Part model, mm, in its own coordinate system. Face numbers are marked on the shaded views. Coordinates: 2 decimals unless noted, no trailing zeros. Order: outer loops, then holes, each group sorted by start corner. A loop starts at its lowest first (then second) coordinate and runs counter-clockwise, first axis right, second up.
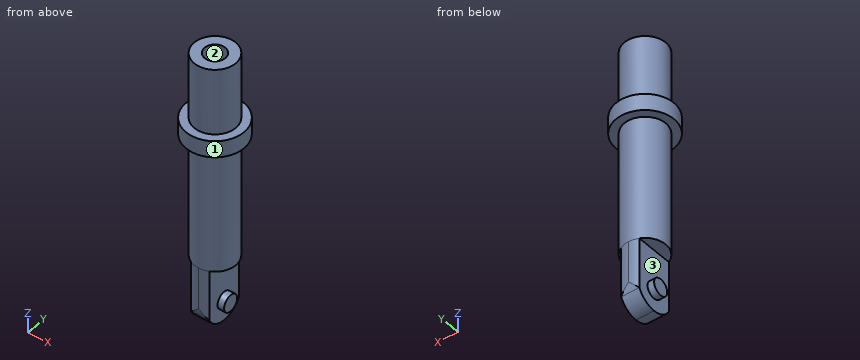
from build123d import *

# Parameters (mm, degrees)
F0_R          = 5
F1_DEPTH      = 50
F3_DEPTH      = 15
F5_DEPTH      = 25
F6_R          = 2
F7_DEPTH      = 1.6
F7_DEPTH_BACK = 6
F8_R          = 2.5
F9_DEPTH      = 10
F11_R         = 7
F11_R_2       = 5
F12_DEPTH     = 4


with BuildPart() as f1:
    # F0 (on Top) → F1 (new body)
    with BuildSketch(Plane.XY):
        Circle(F0_R)
    extrude(amount=F1_DEPTH)

    # F2 (on face) → F3 (join)
    with BuildSketch(Plane(origin=(0, 0, 0), x_dir=(1, 0, 0), z_dir=(0, 0, -1))):
        with BuildLine():
            ThreePointArc((2.2, 4.4899888641), (1.1291713066, 4.8708286934), (0, 5))
            ThreePointArc((0, 5), (-1.1291713066, 4.8708286934), (-2.2, 4.4899888641))
            Line((-2.2, 4.4899888641), (-2.2, -4.4899888641))
            ThreePointArc((-2.2, -4.4899888641), (-1.1291713066, -4.8708286934), (0, -5))
            ThreePointArc((0, -5), (1.1291713066, -4.8708286934), (2.2, -4.4899888641))
            Line((2.2, -4.4899888641), (2.2, 4.4899888641))
        make_face()
    extrude(amount=F3_DEPTH)

    # F4 (on face) → F5 (cut)
    with BuildSketch(Plane.YZ.offset(2.2)):
        with BuildLine():
            Line((5, -15), (5, -10))
            ThreePointArc((5, -10), (4.8708286934, -11.1291713066), (4.4899888641, -12.2))
            Line((4.4899888641, -12.2), (4.4899888641, -15))
            Line((4.4899888641, -15), (5, -15))
        make_face()
        with BuildLine():
            Line((4.4899888641, -15), (4.4899888641, -12.2))
            ThreePointArc((4.4899888641, -12.2), (2.6457513111, -14.2426406871), (0, -15))
            Line((0, -15), (4.4899888641, -15))
        make_face()
        with BuildLine():
            Line((-4.4899888641, -15), (0, -15))
            ThreePointArc((0, -15), (-2.6457513111, -14.2426406871), (-4.4899888641, -12.2))
            Line((-4.4899888641, -12.2), (-4.4899888641, -15))
        make_face()
        with BuildLine():
            ThreePointArc((-4.4899888641, -12.2), (-4.8708286934, -11.1291713066), (-5, -10))
            Line((-5, -10), (-5, -15))
            Line((-5, -15), (-4.4899888641, -15))
            Line((-4.4899888641, -15), (-4.4899888641, -12.2))
        make_face()
    extrude(amount=-F5_DEPTH, mode=Mode.SUBTRACT)

    # F6 (on face) → F7 (join, two sides)
    with BuildSketch(Plane.YZ.offset(2.2)) as f7_sk:
        with Locations((0, -10)):
            Circle(F6_R)
    extrude(amount=F7_DEPTH)
    extrude(f7_sk.sketch, amount=-F7_DEPTH_BACK)

    # F8 (on face) → F9 (cut)
    with BuildSketch(Plane.XY.offset(50)):
        Circle(F8_R)
    extrude(amount=-F9_DEPTH, mode=Mode.SUBTRACT)

    # F11 (on offset) → F12 (join)
    with BuildSketch(Plane.XY.offset(30)):
        Circle(F11_R)
        Circle(F11_R_2, mode=Mode.SUBTRACT)
    extrude(amount=F12_DEPTH)


solid = f1.part
Q1. Wall check: line 1 along Y through (x, z) = (0, 45.5); line 2 along X through (y, z) = (-0.25, 45.5); line 3 along Z through (x, y) = (5.5, 2.25). Give the ranges that are in metal, low to high.
Results list:
line 1: y = -5 to -2.5, 2.5 to 5
line 2: x = -4.99 to -2.49, 2.49 to 4.99
line 3: z = 30 to 34
Q2. Cut at A-A on x = -1.25. Write the cut outline in (y, z), and give its area (3 significant figures).
Results list:
outline: (-6.89, 30) - (-4.84, 30) - (-4.84, -11.25) arc R5 ccw to (4.84, -11.25) - (4.84, 30) - (6.89, 30) - (6.89, 34) - (4.84, 34) - (4.84, 50) - (2.17, 50) - (2.17, 40) - (-2.17, 40) - (-2.17, 50) - (-4.84, 50) - (-4.84, 34) - (-6.89, 34) - close
area: 593 mm2
Q3. Cut at C-C on y = 5.75. Write the cut outline in (x, z).
Results list:
outline: (-3.99, 30) - (3.99, 30) - (3.99, 34) - (-3.99, 34) - close
Q4. Cut at B-B on z = 2. Write the cut outline in (x, y), and give its area (3 significant figures).
Results list:
outline: circle Ø10 at (0, 0)
area: 78.5 mm2
Q5. Mould opens along X. For the marked faces 1, 2 and 3 say: pulls with the +X half, pulls with the -X half, needs draft (parallel to the pull), parting line crosses it, or undercut.
Results list:
face 1: parting line crosses it
face 2: undercut
face 3: pulls with the -X half
Q6. Pin check, flat tips, straight feed: pin 1 Ø4 at (x, z) = (5, 6.5) entering from -Y; pin 2 Ø1.4 at (x, y) = (3.5, 2) entering from -Z; pin 3 Ø3 at (y, z) = (-0.5, -10) entering from +X. Stop position of each tip, or through.
Results list:
pin 1: stops at y = -4
pin 2: stops at z = -11.52
pin 3: stops at x = 3.8
